Model file for the job. Use its own axes, mm. A direction names the side the tool comes from. Round coordinates to 2 decimals unless told otherwise and drop trailing zeros. Order: outer loops, then holes, each group sorted by start corner. A loop starts at its lowest first (then second) coordinate and runs counter-clockwise, first axis right, second up. Notation, with made-up numbers: (55, -1) - (79, -1) arc R19 cw to (79, 30) - close; hole circle Ø10 at (-6, 19). An arc over 180 degrees is marked (long way). Use one line per item in the form item = value.
from build123d import *

# Parameters (mm, degrees)
SKETCH1_W               = 6.01
SKETCH1_H               = 6.01
BOSS_EXTRUDE1_DEPTH     = 3
CHAMFER1_SIZE           = 0.5
SKETCH3_R               = 1.75
BOSS_EXTRUDE2_DEPTH     = 2
SKETCH4_R               = 0.5
BOSS_EXTRUDE6_DEPTH     = 0.5
SKETCH5_R               = 0.5
BOSS_EXTRUDE7_DEPTH     = 0.5
SKETCH6_W               = 0.7
SKETCH6_H               = 0.2
MIRROR2_COPY_1_SKETCH_W = 0.7
MIRROR2_COPY_1_SKETCH_H = 0.2
CUT_EXTRUDE1_DEPTH      = 4.782799277


with BuildPart() as part:
    # Sketch1 → Boss-Extrude1 (new body)
    with BuildSketch(Plane(origin=(0, 0, 0), x_dir=(1, 0, 0), z_dir=(0, 1, 0))):
        Rectangle(SKETCH1_W, SKETCH1_H)
    extrude(amount=BOSS_EXTRUDE1_DEPTH)

    # Chamfer1
    chamfer1_edges = [part.edges().sort_by_distance(p)[0] for p in [
        (3.005, 1.5, 3.005),
        (-3.005, 1.5, 3.005),
        (-3.005, 1.5, -3.005),
        (3.005, 1.5, -3.005),
    ]]
    chamfer(chamfer1_edges, length=CHAMFER1_SIZE)

    # Sketch3 → Boss-Extrude2 (add)
    with BuildSketch(Plane(origin=(0, 3, 0), x_dir=(1, 0, 0), z_dir=(0, 1, 0))):
        Circle(SKETCH3_R)
    extrude(amount=BOSS_EXTRUDE2_DEPTH)

    # Sketch4 → Boss-Extrude6 (add)
    with BuildSketch(Plane(origin=(0, 3, 0), x_dir=(1, 0, 0), z_dir=(0, 1, 0))):
        with Locations((2.25, 2.25)):
            Circle(SKETCH4_R)
        with Locations((2.25, -2.25)):
            Circle(SKETCH4_R)
        with Locations((-2.25, 2.25)):
            Circle(SKETCH4_R)
    extrude(amount=BOSS_EXTRUDE6_DEPTH)

    # Sketch5 → Boss-Extrude7 (add)
    with BuildSketch(Plane(origin=(0, 3, 0), x_dir=(1, 0, 0), z_dir=(0, 1, 0))):
        with Locations((-2.25, -2.25)):
            Circle(SKETCH5_R)
    extrude(amount=BOSS_EXTRUDE7_DEPTH)

    # Sweep1: sweep along a path in Sketch7
    with BuildLine(Plane.XY) as sweep1_path:
        Line((-3.005, 0.9), (-3.105, 0.726794919))
        Line((-3.105, 0.726794919), (-3.105, -0.773205081))
        Line((-3.105, -0.773205081), (-3.72715614, -1.850811126))
        Line((-3.72715614, -1.850811126), (-3.25, -3))
        Line((-3.25, -3), (-3.25, -3.5))
    # Sketch6 → Sweep1 (sweep)
    with BuildSketch(Plane.ZY.offset(3.005)):
        with Locations((-1.955, 0.9)):
            Rectangle(SKETCH6_W, SKETCH6_H)
    sweep1 = sweep(path=sweep1_path.line, transition=Transition.RIGHT)

    # Mirror1: Sweep1 across plane
    add(sweep1.mirror(Plane.XY))

    # Mirror2: Sweep1 across plane
    add(sweep1.mirror(Plane(origin=(0, 0, 0), x_dir=(0, 0, 1), z_dir=(1, 0, 0))))

    # Mirror2 copy 1: sweep along a path in Mirror2 copy 1 path
    with BuildLine(Plane(origin=(0, 0, 0), x_dir=(-1, 0, 0), z_dir=(0, 0, -1))) as mirror2_copy_1_path:
        Line((-3.005, 0.9), (-3.105, 0.726794919))
        Line((-3.105, 0.726794919), (-3.105, -0.773205081))
        Line((-3.105, -0.773205081), (-3.72715614, -1.850811126))
        Line((-3.72715614, -1.850811126), (-3.25, -3))
        Line((-3.25, -3), (-3.25, -3.5))
    # Mirror2 copy 1 sketch → Mirror2 copy 1 (sweep)
    with BuildSketch(Plane(origin=(3.005, 0, 0), x_dir=(0, 0, -1), z_dir=(1, 0, 0))):
        with Locations((-1.955, 0.9)):
            Rectangle(MIRROR2_COPY_1_SKETCH_W, MIRROR2_COPY_1_SKETCH_H)
    sweep(path=mirror2_copy_1_path.line, transition=Transition.RIGHT)

    # Sketch8 → Cut-Extrude1 (cut, symmetric)
    with BuildSketch(Plane(origin=(0, 0, 0), x_dir=(0, 0, -1), z_dir=(1, 0, 0))):
        with BuildLine():
            Line((-2.305, -3.211682602), (-2.305, -3.58660254))
            Line((-2.305, -3.58660254), (-1.605, -3.58660254))
            Line((-1.605, -3.58660254), (-1.605, -3.211682602))
            Line((-1.605, -3.211682602), (-1.881694927, -3.48928466))
            ThreePointArc((-1.881694927, -3.48928466), (-1.952077784, -3.518688814), (-2.022718654, -3.489910032))
            Line((-2.022718654, -3.489910032), (-2.305, -3.211682602))
        make_face()
    cut_extrude1 = extrude(amount=CUT_EXTRUDE1_DEPTH, both=True, mode=Mode.SUBTRACT)

    # Mirror3: Cut-Extrude1 across plane
    add(cut_extrude1.mirror(Plane.XY), mode=Mode.SUBTRACT)


solid = part.part
(1) Slice it at A-A on y = 0.25. Give the cut face in (x, z) (3 decimals), then the cut area to 3 significant figures.
Report:
outline = (-3.155, -2.305) - (-3.055, -2.305) - (-3.055, -1.605) - (-3.155, -1.605) - close; (-3.155, 1.605) - (-3.055, 1.605) - (-3.055, 2.305) - (-3.155, 2.305) - close; (-3.005, -2.505) - (-2.505, -3.005) - (2.505, -3.005) - (3.005, -2.505) - (3.005, 2.505) - (2.505, 3.005) - (-2.505, 3.005) - (-3.005, 2.505) - close; (3.055, -2.305) - (3.155, -2.305) - (3.155, -1.605) - (3.055, -1.605) - close; (3.055, 1.605) - (3.155, 1.605) - (3.155, 2.305) - (3.055, 2.305) - close
area = 35.9 mm2
(2) Tool access for faces 5 (the face through (1.617, 3.986, 0.67)), 6 (the face through (-2.3, 3.5, 2.2)): list every direction of +Z, -Z, +X, -X, +Y, -Y with a clear straight run to the whole face (end or side of a thin tool).
Report:
face_5 = +Y
face_6 = +Z, -Z, +X, -X, +Y
(3) Probe probe 1 along Y at (x, z) = (0, 2.25); probe 2 along X at (y, z) = (0.75, -1.5) (3 decimals); probe 3 along Z at (x, y) = (0, 4). List the from-to ranges inside material, lowest first. Write a range as [from, to].
Report:
probe_1 = [0, 3]
probe_2 = [-3.005, 3.005]
probe_3 = [-1.75, 1.75]
(4) Slice it at C-C on x = 2.25. Give the cut face in (y, z) (3 decimals), then the cut area to 3 significant figures.
Report:
outline = (0, -3.005) - (3, -3.005) - (3, -2.75) - (3.5, -2.75) - (3.5, -1.75) - (3, -1.75) - (3, 1.75) - (3.5, 1.75) - (3.5, 2.75) - (3, 2.75) - (3, 3.005) - (0, 3.005) - close
area = 19.0 mm2
(5) Slice it at B-B on z = 0. Give the cut face in (x, y) (3 decimals), then the cut area to 3 significant figures.
Report:
outline = (-3.005, 0) - (3.005, 0) - (3.005, 3) - (1.75, 3) - (1.75, 5) - (-1.75, 5) - (-1.75, 3) - (-3.005, 3) - close
area = 25.0 mm2
(6) Pin check, flat tips, straight feed: pin 1 (3.5 mm diameter, centred on y = 1, z = -1, fed in from -X) (3 decimals); pin 2 (0.9 mm diameter, centred on x = 3.5, y = -2, fed in from -Z) (3 decimals); pin 3 (0.8 mm diameter, centred on x = 2, z = 2.5, fed in from +Y). Stop position of each tip, or through.
Report:
pin_1 = -3.155
pin_2 = -2.305
pin_3 = 3.5
(7) Slice it at D-D on y = -1.25. Give the cut face in (x, z) (3 decimals).
Report:
outline = (-3.438, -2.305) - (-3.323, -2.305) - (-3.323, -1.605) - (-3.438, -1.605) - close; (-3.438, 1.605) - (-3.323, 1.605) - (-3.323, 2.305) - (-3.438, 2.305) - close; (3.323, -2.305) - (3.438, -2.305) - (3.438, -1.605) - (3.323, -1.605) - close; (3.323, 1.605) - (3.438, 1.605) - (3.438, 2.305) - (3.323, 2.305) - close
(8) Pull direction Z, two halves, no side cores. Call faces 1 (the face through (0, 0, 0)), 2 (the face through (-2.315, 3.246, 1.754)), 3 (the face through (0, 1, -3.005)), 4 (the face through (0, 1, 3.005)): released by +Z, released by -Z, zero draft, split by the parting line, or undercut.
Report:
face_1 = zero draft
face_2 = undercut
face_3 = released by -Z
face_4 = released by +Z
